The listing builds one solid part. Answer for the finished solid, in the listing's coordinates (mm). A direction names the side the tool comes from. Give positions to 0.01 mm unless a question says otherwise; leave off trailing zeros. Write each loop counter-clockwise with the first axis right and the second up, starting at its lowest first coordinate (ties: lowest second). Pieces come first, ordered by that corner, then holes. Notation, with made-up numbers: (8, -31) -> (34, -31) arc R25 ccw to (34, -11) -> close; hole circle Ø4 at (26.5, 7). An arc over 180 degrees is marked (long way). Write each question's results on one line, items separated by ' | '. Start each with the question number.
from build123d import *

# Parameters (mm, degrees)
F0_W     = 165
F0_H     = 28
F1_DEPTH = 7
F2_R     = 3


with BuildPart() as f1:
    # F0 (on Top) → F1 (new body)
    with BuildSketch(Plane.XY):
        Polygon((-8.65, 28), (0, 28), (165, 28), (173.65, 28), (173.65, 35), (-8.65, 35), align=None)
        Polygon((-15.65, 0), (-8.65, 0), (-8.65, 28), (-8.65, 35), (-15.65, 35), align=None)
        Polygon((165, 0), (0, 0), (-8.65, 0), (-15.65, 0), (-15.65, -7), (173.65, -7), (173.65, 0), align=None)
        with Locations((82.5, 14)):
            Rectangle(F0_W, F0_H)
        Polygon((173.65, 28), (173.65, 0), (173.65, -7), (180.65, -7), (180.65, 35), (173.65, 35), align=None)
    extrude(amount=F1_DEPTH)

    # F2
    f2_edges = [f1.edges().sort_by_distance(p)[0] for p in [
        (180.65, -7, 3.5),
        (180.65, 35, 3.5),
        (-15.65, -7, 3.5),
        (-15.65, 35, 3.5),
    ]]
    fillet(f2_edges, radius=F2_R)


solid = f1.part
1. Section A-A (x = -3) is taken. Write down the section's boundary in (y, z).
2. Section B-B (y = 2) is taken. Write down the section's boundary in (x, z).
3. A tool of negligible diameter and unlimited length cuts with its end or side. For faces 5 (the flat face through (-4, 28, 3)), 6 (the flat face through (81, 14, 7)), from which of +Z, -Z, +X, -X, +Y, -Y can it reach the whole face along a straight path? Write none if from no direction.
4. Consider probe 1 along X at (y, z) = (14.5, 1.5); probe 2 along Y at (x, z) = (-6.5, 4.75). Determine where each line is inside the solid, lowest interval first. Write a range as [from, to].
5. Section C-C (z = 2) is taken. Write down the section's boundary in (x, y).
6. The mould has two halves that part along X. Classify faces 1 (the flat face through (-8.65, 14, 3)), 2 (the flat face through (81, -7, 3)), 3 (the flat face through (-15.65, 14, 3)), 4 (the flat face through (180.65, 14, 3)): pulls with the +X half, pulls with the -X half, needs draft (parallel to the pull), parting line crosses it, or undercut.
Results:
1) outline: (-7, 0) -> (0, 0) -> (0, 7) -> (-7, 7) -> close; (28, 0) -> (35, 0) -> (35, 7) -> (28, 7) -> close
2) outline: (-15.65, 0) -> (-8.65, 0) -> (-8.65, 7) -> (-15.65, 7) -> close; (0, 0) -> (165, 0) -> (165, 7) -> (0, 7) -> close; (173.65, 0) -> (180.65, 0) -> (180.65, 7) -> (173.65, 7) -> close
3) face 5: +Z, -Z | face 6: +Z, +X, -X, +Y, -Y
4) probe 1: x = [-15.65, -8.65], [0, 165], [173.65, 180.65] | probe 2: y = [-7, 0], [28, 35]
5) outline: (-15.65, -4) arc R3 ccw to (-12.65, -7) -> (177.65, -7) arc R3 ccw to (180.65, -4) -> (180.65, 32) arc R3 ccw to (177.65, 35) -> (-12.65, 35) arc R3 ccw to (-15.65, 32) -> close; hole (-8.65, 0) -> (0, 0) -> (0, 28) -> (-8.65, 28) -> close; hole (165, 0) -> (173.65, 0) -> (173.65, 28) -> (165, 28) -> close
6) face 1: undercut | face 2: needs draft | face 3: pulls with the -X half | face 4: pulls with the +X half
